The drawing under review shows one solid part. Ordinate dimensions are in mm from its lowest x, y, z. A direction names the side the tool comes from. Round coordinates to 2 decimals unless told otherwise and drop trailing zeros. Write each loop counter-clockwise with the first axis right and the second up, starting at its lowest first coordinate (ties: lowest second). Pieces come first, ordered by that corner, then holes.
Item 1: Add section A-A (x = 1.05). Give the boundary of the cut face in (y, z).
Item 2: Add section C-C (y = 5.75). Give the boundary of the cut face in (x, z) (1 decimal), plus the area to 3 significant figures.
Item 3: Add section D-D (z = 10.25). Give the boundary of the cut face in (x, y).
Item 4: Machinability: for the marked faces 1 and 2, which of the approach directions +Z, -Z, +X, -X, +Y, -Y give a long, thin tool a straight path to every point of the face, cutting with its end or side? Answer none if there is none.
Item 5: Add section B-B (z = 5.5). Give the boundary of the cut face in (x, y).
Item 6: Clearance check with a flat-ended pin moving along its axis: pin 1 Ø4 at (y, z) = (5.5, 9.5) entering from -X. State where the tip first meets the part, or that it passes through.
Item 7: Draft analysis for pull direction Y (two halves, no side actions). For the marked faces 3, 4 and 5, state which applies: +Y half, -Y half, draft (parallel to the pull), parting line (faces both ways), or undercut.
Item 8: To check wall thickness, follow L1, parallel to Y at x = 2.4, z = 7.25 (1 decimal); L2, parallel to Z at x = 1.6, y = 5.25 (1 decimal); L3, parallel to Z at x = 1.2, y = 6. State the ranges of each line that lie inside material, in increasing order.
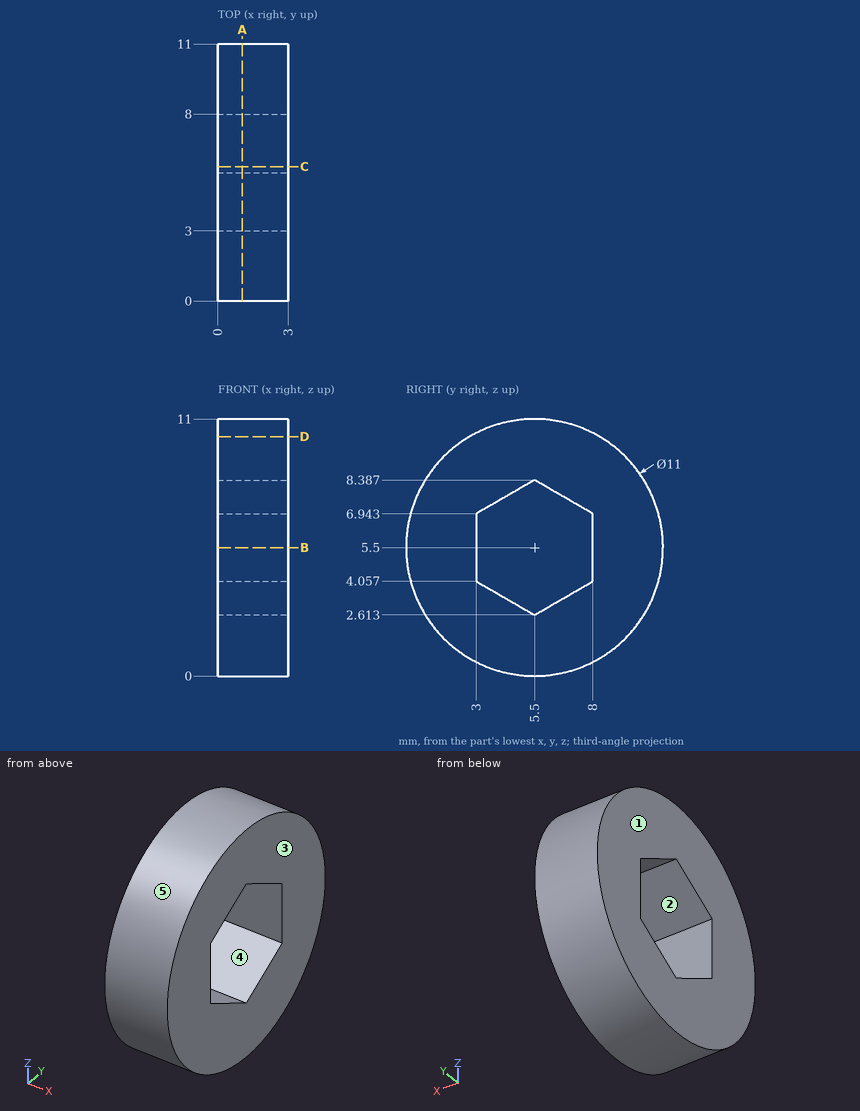
Numbers:
1. outline: circle Ø11 at (5.5, 5.5); hole (3, 4.06) - (5.5, 2.61) - (8, 4.06) - (8, 6.94) - (5.5, 8.39) - (3, 6.94) - close
2. outline: (0, 0) - (3, 0) - (3, 2.8) - (0, 2.8) - close; (0, 8.2) - (3, 8.2) - (3, 11) - (0, 11) - close
2. area: 16.5 mm2
3. outline: (0, 2.73) - (3, 2.73) - (3, 8.27) - (0, 8.27) - close
4. face 1: +Z, -Z, -X, +Y, -Y
4. face 2: +X, -X
5. outline: (0, 0) - (3, 0) - (3, 3) - (0, 3) - close; (0, 8) - (3, 8) - (3, 11) - (0, 11) - close
6. pin 1: stops at x = 0
7. face 3: draft
7. face 4: undercut
7. face 5: parting line
8. L1: y = 0.3 to 3.5, 7.5 to 10.7
8. L2: z = 0 to 2.8, 8.2 to 11
8. L3: z = 0.02 to 2.9, 8.1 to 10.98
